```python
from build123d import *

# Parameters (mm, degrees)
BOSS_EXTRUDE1_DEPTH = 25
SKETCH2_R           = 37.75
CUT_EXTRUDE1_DEPTH  = 28
SKETCH3_R           = 7
CUT_EXTRUDE2_DEPTH  = 173.13028653


with BuildPart() as part:
    # Sketch1 → Boss-Extrude1 (new body)
    with BuildSketch(Plane(origin=(0, 0, 0), x_dir=(1, 0, 0), z_dir=(0, 1, 0))):
        with BuildLine():
            Line((66.645984298, 85.104941493), (128.643951995, -22.278688525))
            ThreePointArc((128.643951995, -22.278688525), (128.643951995, -62.278688525), (94.002935844, -82.278688525))
            Line((94.002935844, -82.278688525), (-29.992999551, -82.278688525))
            ThreePointArc((-29.992999551, -82.278688525), (-64.634015702, -62.278688525), (-64.634015702, -22.278688525))
            Line((-64.634015702, -22.278688525), (-2.636048005, 85.104941493))
            ThreePointArc((-2.636048005, 85.104941493), (32.004968146, 105.104941493), (66.645984298, 85.104941493))
        make_face()
    extrude(amount=BOSS_EXTRUDE1_DEPTH)

    # Sketch2 → Cut-Extrude1 (cut)
    with BuildSketch(Plane(origin=(0, 25, 0), x_dir=(1, 0, 0), z_dir=(0, 1, 0))):
        with Locations(Location((32.004968146, -4.752094378, 0), (0, 0, 270))):
            Circle(SKETCH2_R)
    extrude(amount=-CUT_EXTRUDE1_DEPTH, mode=Mode.SUBTRACT)

    # Sketch3 → Cut-Extrude2 (cut, through all)
    with BuildSketch(Plane(origin=(0, 25, 0), x_dir=(1, 0, 0), z_dir=(0, 1, 0))):
        with Locations(Location((32.004968146, 84.737197347, 0), (0, 0, 270))):
            Circle(SKETCH3_R)
        with Locations(Location((109.504968146, -49.49674024, 0), (0, 0, 270))):
            Circle(SKETCH3_R)
        with Locations(Location((-45.495031854, -49.49674024, 0), (0, 0, 270))):
            Circle(SKETCH3_R)
    extrude(amount=-CUT_EXTRUDE2_DEPTH, mode=Mode.SUBTRACT)


solid = part.part
```
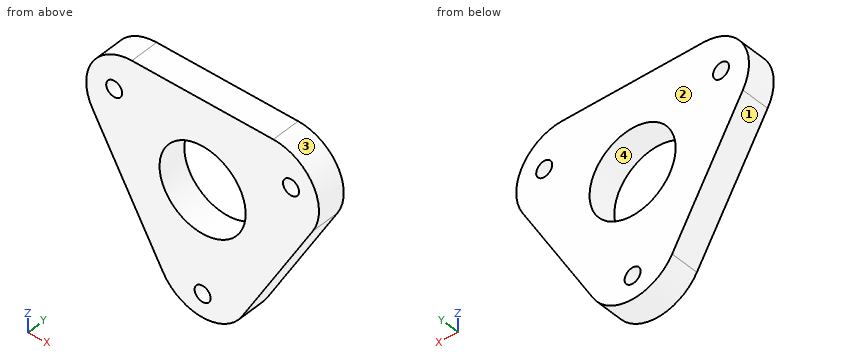
The listing builds one solid part. Answer for the finished solid, in the listing's coordinates (mm). Face numbers are marked on the shaded views. Give positions to 0.01 mm unless a question says otherwise; leave off trailing zeros. Order: outer loops, then holes, each group sorted by start corner. A loop starts at its lowest first (then second) coordinate and runs counter-clockwise, first axis right, second up. Notation, with made-up numbers: (6, 17) -> (56, 17) arc R20 ccw to (56, 30) -> close; hole circle Ø1 at (-37.75, -11.75). An arc over 180 degrees is marked (long way). Answer as a JSON object with one key per item and string values. Group by question number.
Item 1: Flat-ended cylindrical pins translate along their axes: pin 1 (6 mm diameter, centred on y = 8, z = -3, fed in from +X); pin 2 (3 mm diameter, centred on x = 52.5, y = 14, fed in from -Z); pin 3 (1.5 mm diameter, centred on y = 17.5, z = 14.5, fed in from +X); pin 4 (8.5 mm diameter, centred on x = 109.5, z = 49.5, fed in from -Y). Find the tip coordinate at first contact, or state that the pin passes through.
Item 2: Determine the mould class of the marked faces 1, 2, 3 and 4 for opening direction Z: pulls with the +Z half, pulls with the -Z half, needs draft (parallel to the pull), parting line crosses it, or undercut.
Item 3: The part is cut by section B-B on z = -89. Write down the section's boundary in (x, y).
Item 4: Consider L1, parallel to Z at x = 104, y = 3.75; L2, parallel to X at y = 20, z = 12.5; L3, parallel to Z at x = 107.5, y = 15.5. Determine where each line is inside the solid, lowest interval first. Write a range as from..to.
Item 5: The part is cut by section D-D on z = 50. Write down the section's boundary in (x, y), and give its area (3 significant figures).
Item 6: The part is cut by section C-C on y = 16.5. Write down the section's boundary in (x, z).
Item 7: The part is cut by section A-A on x = 3.5. Write down the section's boundary in (y, z), and give its area (3 significant figures).
Result set:
{
 "1": {"pin 1": "x = 115.78", "pin 2": "z = -100.31", "pin 3": "x = 124.59", "pin 4": "through"},
 "2": {"face 1": "pulls with the -Z half", "face 2": "needs draft", "face 3": "parting line crosses it", "face 4": "undercut"},
 "3": {"outline": "(-0.07, 0) -> (26.45, 0) -> (26.45, 25) -> (-0.07, 25) -> close; (37.56, 0) -> (64.08, 0) -> (64.08, 25) -> (37.56, 25) -> close"},
 "4": {"L1": "-20.41..45.17, 53.82..81.01", "L2": "-58.99..-4.94, 68.95..123", "L3": "-14.34..42.79, 56.2..79.93"},
 "5": {"outline": "(-69.24, 0) -> (-52.48, 0) -> (-52.48, 25) -> (-69.24, 25) -> close; (-38.51, 0) -> (102.52, 0) -> (102.52, 25) -> (-38.51, 25) -> close; (116.49, 0) -> (133.25, 0) -> (133.25, 25) -> (116.49, 25) -> close", "area": "4,360 mm²"},
 "6": {"outline": "(-64.63, 22.28) -> (-2.64, -85.1) arc R40 ccw to (66.65, -85.1) -> (128.64, 22.28) arc R40 ccw to (94, 82.28) -> (-29.99, 82.28) arc R40 ccw to start; hole circle Ø14 at (-45.5, 49.5); hole circle Ø75.5 at (32, 4.75); hole circle Ø14 at (32, -84.74); hole circle Ø14 at (109.5, 49.5)"},
 "7": {"outline": "(0, -93.17) -> (25, -93.17) -> (25, -20) -> (0, -20) -> close; (0, 29.5) -> (25, 29.5) -> (25, 82.28) -> (0, 82.28) -> close", "area": "3,150 mm²"}
}
